```python
from build123d import *

# Parameters (mm, degrees)
SKETCH2_W           = 50.8
SKETCH2_H           = 35.56
SKETCH2_R           = 3.2639
BOSS_EXTRUDE1_DEPTH = 39.37
SKETCH4_R           = 4.9022
CUT_EXTRUDE1_DEPTH  = 59.818963779
SKETCH5_W           = 50.8
SKETCH5_H           = 20.6502
CUT_EXTRUDE2_DEPTH  = 33.02


with BuildPart() as part:
    # Sketch2 → Boss-Extrude1 (new body)
    with BuildSketch(Plane(origin=(0, 0, 0), x_dir=(1, 0, 0), z_dir=(0, 1, 0))):
        Rectangle(SKETCH2_W, SKETCH2_H)
        with Locations(Location((-16.51, 0, 0), (0, 0, 270))):
            Circle(SKETCH2_R, mode=Mode.SUBTRACT)
        with Locations(Location((16.51, 0, 0), (0, 0, 90))):
            Circle(SKETCH2_R, mode=Mode.SUBTRACT)
    extrude(amount=-BOSS_EXTRUDE1_DEPTH)

    # Sketch4 → Cut-Extrude1 (cut, through all)
    with BuildSketch(Plane.XY.offset(17.78)):
        with Locations((0, -30.196811844)):
            Circle(SKETCH4_R)
        Polygon((-25.4, -6.35), (-6.35, -39.37), (-25.4, -39.37), align=None)
        Polygon((6.35, -39.37), (25.4, -39.37), (25.4, -6.35), align=None)
    extrude(amount=-CUT_EXTRUDE1_DEPTH, mode=Mode.SUBTRACT)

    # Sketch5 → Cut-Extrude2 (cut)
    with BuildSketch(Plane.XZ.offset(39.37)):
        Rectangle(SKETCH5_W, SKETCH5_H)
    extrude(amount=-CUT_EXTRUDE2_DEPTH, mode=Mode.SUBTRACT)


solid = part.part
```
Design review of the part built by this model. Coordinates are the model's own, in mm. A direction names the side the tool comes from. Give positions to 0.01 mm unless a question says otherwise; leave off trailing zeros. Write each loop counter-clockwise with the first axis right and the second up, starting at its lowest first coordinate (ties: lowest second). Pieces come first, ordered by that corner, then holes. Notation, with made-up numbers: (4, -5) - (15, -5) arc R26 ccw to (15, 15) - close; hole circle Ø3 at (66.5, 13.5). An arc over 180 degrees is marked (long way). Return JSON: item names as keys, results as strings. Group by question number.
(1) To check wall thickness, follow probe 1 along X at (y, z) = (-3.5, 0); probe 2 along Z at (x, y) = (9, -23.5); probe 3 along Y at (x, z) = (0, 13). State the ranges of each line that lie inside material, in increasing order.
(2) We need section A-A, the plane x = 0. Give the boundary of the cut face in (y, z).
(3) We need section C-C, the plane y = -15. Give the boundary of the cut face in (x, z), then the cut area to 3 significant figures.
(4) We need section B-B, the plane z = 0. Give the boundary of the cut face in (x, y), then the cut area to 3 significant figures.
(5) We need section D-D, the plane z = -14.5. Give the boundary of the cut face in (x, y), then the cut area to 3 significant figures.
(6) Insertion check: pin 1 (6 mm diameter, centred on y = -24.5, z = 14, fed in from -X); pin 2 (5 mm diameter, centred on y = -10.5, z = -10.5, fed in from -X); pin 3 (6 mm diameter, centred on x = -9, z = 3.5, fed in from -Y). Each pin has a flat end and moves straight along its axis. Give the tip position at first contact, or say it passes through.
(7) Mouldability with a two-part tool opening along Y and no side actions: class faces 3 (the flat face through (0, -6.35, 0)), 4 (the cylindrical face through (13.274, -3.131, 0.425)), 5 (the cylindrical face through (-1.063, -34.982, -14)) as +Y half, -Y half, draft (parallel to the pull), parting line (faces both ways), or undercut.
(8) Machinability: for faces 1 (the flat face through (0, -19, 10.325)), 2 (the cylindrical face through (-1.063, -34.982, 14.105)), which of the approach directions +Z, -Z, +X, -X, +Y, -Y give a long, thin tool a straight path to every point of the face, cutting with its end or side? Answer none if there is none.
Reported:
{
 "1": {"probe 1": "x = -25.4 to -19.77, -13.25 to 13.25, 19.77 to 25.4", "probe 2": "z = -17.78 to -10.33, 10.33 to 17.78", "probe 3": "y = -39.37 to -35.1, -25.29 to 0"},
 "2": {"outline": "(-39.37, -17.78) - (-35.1, -17.78) - (-35.1, -10.33) - (-39.37, -10.33) - close; (-39.37, 10.33) - (-35.1, 10.33) - (-35.1, 17.78) - (-39.37, 17.78) - close; (-25.29, -17.78) - (0, -17.78) - (0, 17.78) - (-25.29, 17.78) - (-25.29, 10.33) - (-6.35, 10.33) - (-6.35, -10.33) - (-25.29, -10.33) - close"},
 "3": {"outline": "(-20.41, -17.78) - (20.41, -17.78) - (20.41, -10.33) - (-20.41, -10.33) - close; (-20.41, 10.33) - (20.41, 10.33) - (20.41, 17.78) - (-20.41, 17.78) - close", "area": "609 mm2"},
 "4": {"outline": "(-25.4, -6.35) - (-19.77, -6.35) - (-19.77, 0) - (-25.4, 0) - close; (-13.25, -6.35) - (13.25, -6.35) - (13.25, 0) - (-13.25, 0) - close; (19.77, -6.35) - (25.4, -6.35) - (25.4, 0) - (19.77, 0) - close", "area": "240 mm2"},
 "5": {"outline": "(-25.4, -6.35) - (-6.35, -39.37) - (6.35, -39.37) - (25.4, -6.35) - (25.4, 0) - (-25.4, 0) - close; hole circle Ø9.8 at (0, -30.2)", "area": "1,300 mm2"},
 "6": {"pin 1": "stops at x = -16.66", "pin 2": "stops at x = -24.45", "pin 3": "stops at y = -6.35"},
 "7": {"face 3": "-Y half", "face 4": "draft", "face 5": "undercut"},
 "8": {"face 1": "+X, -X, -Y", "face 2": "+Z, -Z"}
}
